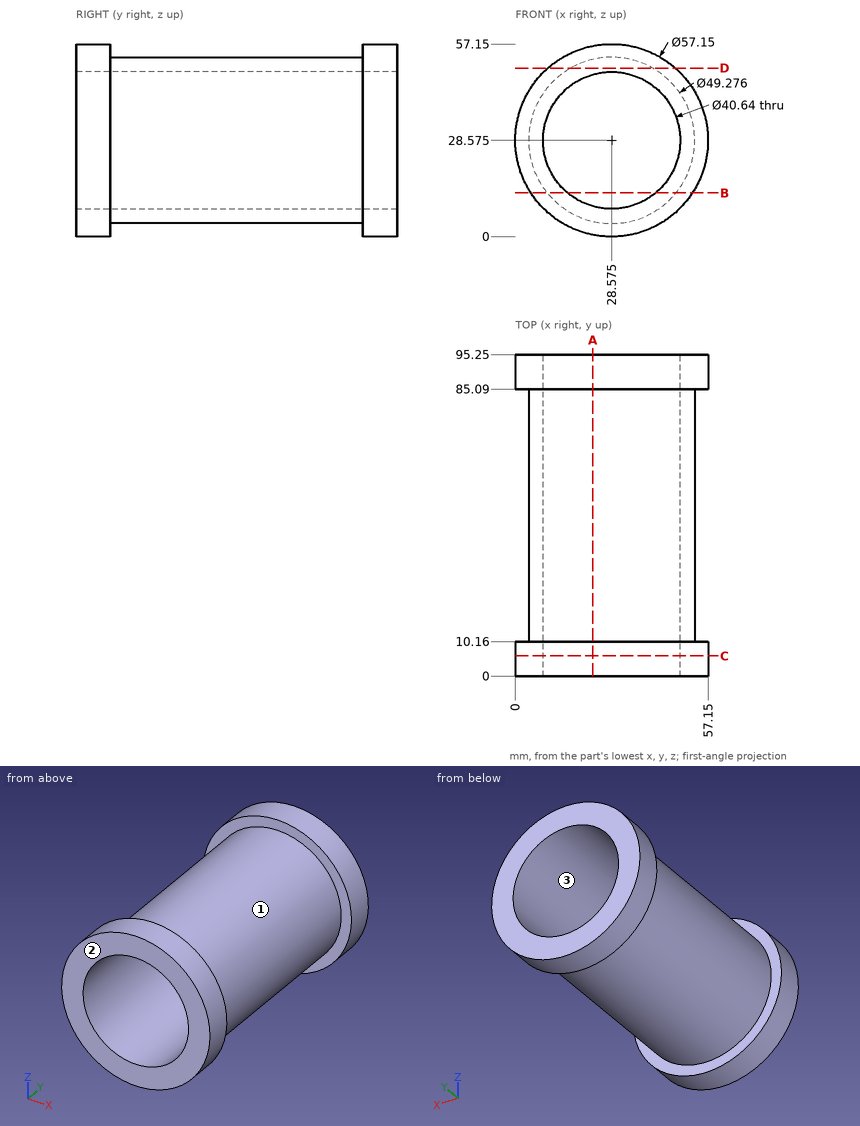
Verification items for this drawing (mm, ordinates from the low corner). Round coordinates to 2 decimals unless told otherwise and drop trailing zeros. Loops run counter-clockwise (first coordinate to the right, second up) from the corner with the lowest first, then second, coordinate; pieces in that order, holes last. Notation, with made-up numbers: (-10, 23.5) -> (20, 23.5) arc R24 ccw to (20, 37.5) -> close; hole circle Ø10 at (35.25, -33). An arc over 180 degrees is marked (long way). Answer in a Markdown table with one row per item.
Q1. Sectioned sample at D-D on z = 50. Enter the section's corners in (x, y), then the cut area to 3 significant figures.
Data:
| item | result |
|---|---|
| outline | (9.67, 0) -> (47.48, 0) -> (47.48, 10.16) -> (40.74, 10.16) -> (40.74, 85.09) -> (47.48, 85.09) -> (47.48, 95.25) -> (9.67, 95.25) -> (9.67, 85.09) -> (16.41, 85.09) -> (16.41, 10.16) -> (9.67, 10.16) -> close |
| area | 2,590 mm^2 |
Q2. Go/stop test with flat-tipped pins: P1, Ø3, axis at x = 17.5, y = 22, coming from the -Z side; P2, Ø1.5, axis at x = 32.5, y = 75.5, coming from the +Z side; P3, Ø6, axis at x = 41, y = 75.5, coming from the +Z side. Record where each tip stops, or that it passes through.
Data:
| item | result |
|---|---|
| P1 | stops at z = 5.87 |
| P2 | stops at z = 53.01 |
| P3 | stops at z = 51.34 |
Q3. Sectioned sample at A-A on x = 23. Enter the section's corners in (y, z), then the cut area to 3 significant figures.
Data:
| item | result |
|---|---|
| outline | (0, 0.55) -> (10.16, 0.55) -> (10.16, 4.58) -> (85.09, 4.58) -> (85.09, 0.55) -> (95.25, 0.55) -> (95.25, 9.03) -> (0, 9.03) -> close; (0, 48.12) -> (95.25, 48.12) -> (95.25, 56.6) -> (85.09, 56.6) -> (85.09, 52.57) -> (10.16, 52.57) -> (10.16, 56.6) -> (0, 56.6) -> close |
| area | 1,010 mm^2 |
Q4. Release check for a two-part mould opening along X. For the marked faces 1, 2 and 3 record: released by +X, released by -X, zero draft, split by the parting line, or undercut.
Data:
| item | result |
|---|---|
| face 1 | split by the parting line |
| face 2 | zero draft |
| face 3 | undercut |
Q5. Sectioned sample at C-C on y = 6. Enter the section's corners in (x, z) (3 decimals).
Data:
| item | result |
|---|---|
| outline | circle Ø57.15 at (28.575, 28.575); hole circle Ø40.64 at (28.575, 28.575) |
Q6. Sectioned sample at B-B on z = 13. Enter the section's corners in (x, y), then the cut area to 3 significant figures.
Data:
| item | result |
|---|---|
| outline | (4.62, 0) -> (15.52, 0) -> (15.52, 95.25) -> (4.62, 95.25) -> (4.62, 85.09) -> (9.48, 85.09) -> (9.48, 10.16) -> (4.62, 10.16) -> close; (41.63, 0) -> (52.53, 0) -> (52.53, 10.16) -> (47.67, 10.16) -> (47.67, 85.09) -> (52.53, 85.09) -> (52.53, 95.25) -> (41.63, 95.25) -> close |
| area | 1,350 mm^2 |
Q7. Thickness scan on L1, parallel to Y at x = 5, z = 43; L2, parallel to X at y = 67, z = 28; L3, parallel to X at y = 58, z = 19.5. Record the ranges inside material, lowest first.
Data:
| item | result |
|---|---|
| L1 | y = 0 to 10.16, 85.09 to 95.25 |
| L2 | x = 3.94 to 8.26, 48.89 to 53.21 |
| L3 | x = 5.67 to 10.39, 46.76 to 51.48 |
